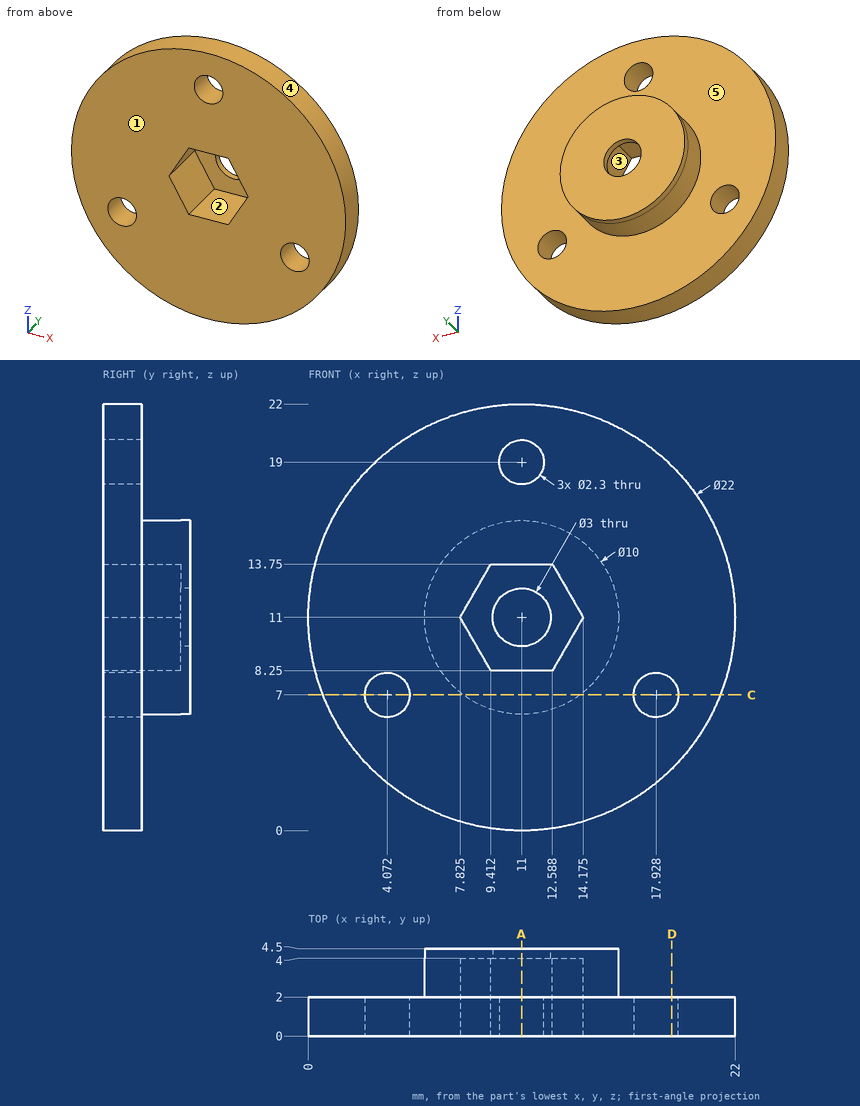
The drawing under review shows one solid part. Ordinate dimensions are in mm from its lowest x, y, z. A direction names the side the tool comes from. Round coordinates to 2 decimals unless told otherwise and drop trailing zeros. Write each loop counter-clockwise with the first axis right and the second up, starting at its lowest first coordinate (ties: lowest second). Pieces come first, ordered by that corner, then holes. Notation, with made-up numbers: (32, -0.75) - (44, -0.75) arc R27 cw to (44, 17.25) - close; hole circle Ø1 at (-8.5, 61). An arc over 180 degrees is marked (long way). Use a Markdown table: item, result. Add a question column.
1. Clearance check with flat-ended pins moving along their axes: pin 1 (2 mm diameter, centred on x = 17.5, y = 0.5, fed in from +Z); pin 2 (6 mm diameter, centred on x = 12.5, z = 11.5, fed in from -Y); pin 3 (2.5 mm diameter, centred on x = 4.07, z = 7, fed in from +Y). State where each tip first meets the part, or that it passes through.
2. We need section C-C (z = 7). State the section outline as (x, y) points.
3. For the marked faces 1 and 2, list the 3-axis set-ups (+Z, -Z, +X, -X, +Y, -Y) from which the entire face can be reached by the end or side of a thin tool; tool diameter is ignored.
4. Wall thickness on probe 1 along Z at (x, y) = (11, 0.8); probe 2 along Z at (x, y) = (11, 4.3); probe 3 along X at (y, z) = (1.75, 7): over which ranges is each line inside the solid? List them lowest first.
5. We need section A-A (x = 11). State the section outline as (y, z) points, then the cut area to 3 significant figures.
6. Mouldability with a two-part tool opening along X and no side actions: class the marked faces 3, 4 and 5 as +X half, -X half, draft (parallel to the pull), parting line (faces both ways), or undercut.
7. We need section D-D (x = 18.75). State the section outline as (y, z) points (1 decimal).
Output:
| question | item | result |
|---|---|---|
| 1 | pin 1 | stops at z = 20.53 |
| 1 | pin 2 | stops at y = 0 |
| 1 | pin 3 | stops at y = 2 |
| 2 | outline | (0.75, 0) - (2.92, 0) - (2.92, 2) - (0.75, 2) - close; (5.22, 0) - (16.78, 0) - (16.78, 2) - (14, 2) - (14, 4.5) - (8, 4.5) - (8, 2) - (5.22, 2) - close; (19.08, 0) - (21.25, 0) - (21.25, 2) - (19.08, 2) - close |
| 3 | face 1 | +Z, -Z, +X, -X, -Y |
| 3 | face 2 | -Y |
| 4 | probe 1 | z = 0 to 8.25, 13.75 to 17.85, 20.15 to 22 |
| 4 | probe 2 | z = 6 to 9.5, 12.5 to 16 |
| 4 | probe 3 | x = 0.75 to 2.92, 5.22 to 16.78, 19.08 to 21.25 |
| 5 | outline | (0, 0) - (2, 0) - (2, 6) - (4.5, 6) - (4.5, 9.5) - (4, 9.5) - (4, 8.25) - (0, 8.25) - close; (0, 13.75) - (4, 13.75) - (4, 12.5) - (4.5, 12.5) - (4.5, 16) - (2, 16) - (2, 17.85) - (0, 17.85) - close; (0, 20.15) - (2, 20.15) - (2, 22) - (0, 22) - close |
| 5 | area | 40.9 mm2 |
| 6 | face 3 | undercut |
| 6 | face 4 | parting line |
| 6 | face 5 | draft |
| 7 | outline | (0, 3.2) - (2, 3.2) - (2, 6.2) - (0, 6.2) - close; (0, 7.8) - (2, 7.8) - (2, 18.8) - (0, 18.8) - close |
